Answer from the drawing. Dimensions are ordinates in mm from the lowest x, y and z of the part. Coordinates: 2 decimals unless noted, no trailing zeros. Loops run counter-clockwise (first coordinate to the right, second up) from the corner with the lowest first, then second, coordinate; pieces in that order, holes last.
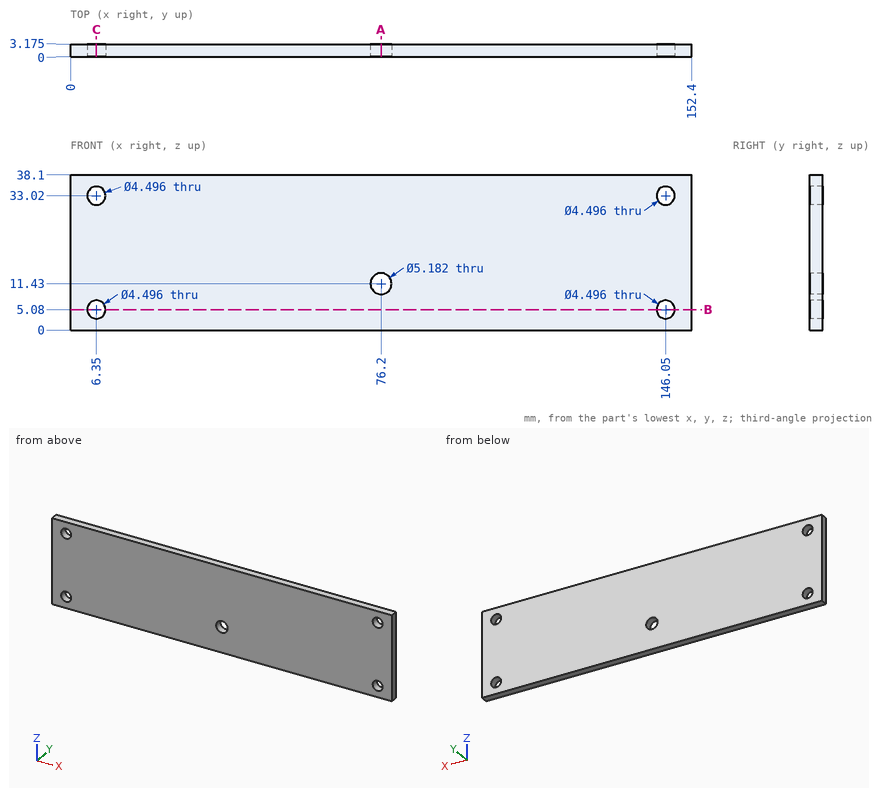
Item 1: A cutting plane is placed at B-B on z = 5.08. Determine the outline of the cut face in (x, y) (1 decimal).
Numbers:
outline: (0, 0) - (4.1, 0) - (4.1, 3.2) - (0, 3.2) - close; (8.6, 0) - (143.8, 0) - (143.8, 3.2) - (8.6, 3.2) - close; (148.3, 0) - (152.4, 0) - (152.4, 3.2) - (148.3, 3.2) - close
Item 2: A cutting plane is placed at A-A on x = 76.2. Determine the outline of the cut face in (y, z) (1 decimal).
Numbers:
outline: (0, 0) - (3.2, 0) - (3.2, 8.8) - (0, 8.8) - close; (0, 14) - (3.2, 14) - (3.2, 38.1) - (0, 38.1) - close
Item 3: Find the intervals of material crossed by line 1 along Z through (x, y) = (6.35, 1.75); line 2 along Z through (x, y) = (76.2, 0.75); line 3 along Z through (x, y) = (8, 2.6) (1 decimal), in increasing order.
Numbers:
line 1: z = 0 to 2.83, 7.33 to 30.77, 35.27 to 38.1
line 2: z = 0 to 8.84, 14.02 to 38.1
line 3: z = 0 to 3.6, 6.6 to 31.5, 34.5 to 38.1
Item 4: A cutting plane is placed at C-C on x = 6.35. Determine the outline of the cut face in (y, z) (1 decimal).
Numbers:
outline: (0, 0) - (3.2, 0) - (3.2, 2.8) - (0, 2.8) - close; (0, 7.3) - (3.2, 7.3) - (3.2, 30.8) - (0, 30.8) - close; (0, 35.3) - (3.2, 35.3) - (3.2, 38.1) - (0, 38.1) - close
Item 5: Given pin 1 (5 mm diameter, centred on x = 146.05, z = 5.08, fed in from -Y); pin 2 (3.5 mm diameter, centred on x = 146.05, z = 33.02, fed in from +Y), each flat-ended and moving along its own axis, determine where each tip first touches the part or whether it passes through.
Numbers:
pin 1: stops at y = 0
pin 2: passes through
